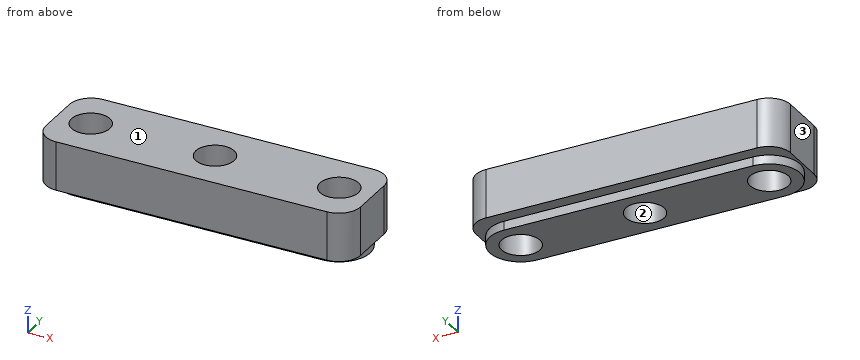
Autodesk Inventor part; units mm, degrees
ref_plane "YZ Plane" through (0, 0, 0) normal (1, 0, 0) x (0, 1, 0)
ref_plane "XZ Plane" through (0, 0, 0) normal (0, 1, 0) x (-1, 0, 0)
ref_plane "XY Plane" through (0, 0, 0) normal (0, 0, 1) x (1, 0, 0)
sketch "Sketch1" plane through (0, 0, 0) normal (0, 0, 1) x (1, 0, 0)
  circle A0 centre (-40.5918, 0) radius 2.4892 construction
  circle A1 centre (-22.5168, 0) radius 2.4892 construction
  circle A2 centre (-4.4418, 0) radius 2.4892 construction
  circle A3 centre (-40.5918, 0) radius 4.5
  circle A4 centre (-4.4418, 0) radius 4.5
  line L0 (-40.5918, 4.5) -> (-4.4418, 4.5)
  line L1 (-4.4418, 4.5) -> (-4.4418, -4.5)
  line L2 (-4.4418, -4.5) -> (-40.5918, -4.5)
  line L3 (-40.5918, -4.5) -> (-40.5918, 4.5)
  point P0 (0, 0)
  dimension "d1" = 9
extrude "Extrusion1" add sketch "Sketch1" along normal blind 1.3
sketch "Sketch2" plane through (0, 0, 1.3) normal (0, 0, 1) x (1, 0, 0)
  line L0 (-45.4068, 6.375) -> (0.3732, 6.375)
  line L1 (0.3732, 6.375) -> (0.3732, -6.375)
  line L2 (0.3732, -6.375) -> (-45.4068, -6.375)
  line L3 (-45.4068, -6.375) -> (-45.4068, 6.375)
  circle A0 centre (-22.5168, 0) radius 2.4892 construction
  point P0 (0, 0)
  dimension "d4" = 45.78
  dimension "d5" = 22.89
  dimension "d6" = 12.75
  dimension "d7" = 6.375
extrude "Extrusion2" add sketch "Sketch2" along normal blind 7.1
fillet "Fillet1" radius 3.175 4 edges at (-45.4068, 6.375, 4.85) (-45.4068, -6.375, 4.85) (0.3732, 6.375, 4.85) (0.3732, -6.375, 4.85)
sketch "Sketch3" plane through (0, 0, 0) normal (0, 0, -1) x (-1, 0, 0)
  circle A0 centre (4.4418, 0) radius 2.4892 construction
  circle A1 centre (22.5168, 0) radius 2.4892 construction
  circle A2 centre (40.5918, 0) radius 2.4892 construction
  circle A3 centre (4.4418, 0) radius 2.794
  circle A4 centre (22.5168, 0) radius 2.794
  circle A5 centre (40.5918, 0) radius 2.794
  point P0 (0, 0)
  dimension "d11" = 5.588
extrude "Extrusion3" cut sketch "Sketch3" against normal through all
equation "\"d5\" = 0.5 * d4"
equation "\"d7\" = 0.5 * d6"
properties part number "NerfBottomStandoff"
Geometry: final body of the model. Coordinates: model frame, mm. Face numbers are marked on the shaded views. Round coordinates to 2 decimals unless told otherwise and drop trailing zeros. Order: outer loops, then holes, each group sorted by start corner. A loop starts at its lowest first (then second) coordinate and runs counter-clockwise, first axis right, second up. Notation, with made-up numbers: M -16,-26 L 16,-26 A28 cw 16,12 Z; hole C -11,-37 d7. An arc over 180 degrees is marked long. Use one line per item in the form item = value. Start each with the question number.
Q1. Material intervals for line 1 (Z direction, x = -5, y = 5.5); line 2 (Y direction, x = -25, z = 6) (3 decimals); line 3 (Y direction, x = -4.5, z = 8.25) (3 decimals), sorted ascending. Write a range as [from, to].
Q2. Cut plane D-D (y = 2). Return loops of the section in (x, z).
Q3. Cut plane A-A (y = 0). Return loops of the section in (x, z), and give its area (3 significant figures).
Q4. Cut plane B-B (z = 6.75). Return loops of the section in (x, y) (3 decimals), and give its area (3 significant figures).
Q5. Cut plane C-C (x = -26). Return loops of the section in (y, z) (3 decimals), and give its area (3 significant figures).
Q6. Pin query (flat end, axial travel): pin 1 Ø1 at (x, z) = (-17.5, 0.5) entering from -Y. Return the tip coordinate at first contact, or that it passes through.
Q7. Mould query, pull axis X, two halves, no side actions, for the marked faces 1, 2 and 3. Classes: +X half, -X half, draft (parallel to the pull), parting line (faces both ways), or undercut.
Geometry results:
q1.line_1 = [1.3, 8.4]
q1.line_2 = [-6.375, -1.281], [1.281, 6.375]
q1.line_3 = [-6.375, -2.793], [2.793, 6.375]
q2.outline = M -45.41,1.3 L -44.62,1.3 L -44.62,0 L -42.54,0 L -42.54,8.4 L -45.41,8.4 Z; M -38.64,0 L -24.47,0 L -24.47,8.4 L -38.64,8.4 Z; M -20.57,0 L -6.39,0 L -6.39,8.4 L -20.57,8.4 Z; M -2.49,0 L -0.41,0 L -0.41,1.3 L 0.37,1.3 L 0.37,8.4 L -2.49,8.4 Z
q3.outline = M -45.41,1.3 L -45.09,1.3 L -45.09,0 L -43.39,0 L -43.39,8.4 L -45.41,8.4 Z; M -37.8,0 L -25.31,0 L -25.31,8.4 L -37.8,8.4 Z; M -19.72,0 L -7.24,0 L -7.24,8.4 L -19.72,8.4 Z; M -1.65,0 L 0.06,0 L 0.06,1.3 L 0.37,1.3 L 0.37,8.4 L -1.65,8.4 Z
q3.area = 243 mm^2
q4.outline = M -45.407,-3.2 A3.175 ccw -42.232,-6.375 L -2.802,-6.375 A3.175 ccw 0.373,-3.2 L 0.373,3.2 A3.175 ccw -2.802,6.375 L -42.232,6.375 A3.175 ccw -45.407,3.2 Z; hole C -40.592,0 d5.588; hole C -22.517,0 d5.588; hole C -4.442,0 d5.588
q4.area = 501 mm^2
q5.outline = M -6.375,1.3 L -4.5,1.3 L -4.5,0 L 4.5,0 L 4.5,1.3 L 6.375,1.3 L 6.375,8.4 L -6.375,8.4 Z
q5.area = 102 mm^2
q6.pin_1 = -4.5
q7.face_1 = draft
q7.face_2 = undercut
q7.face_3 = -X half
